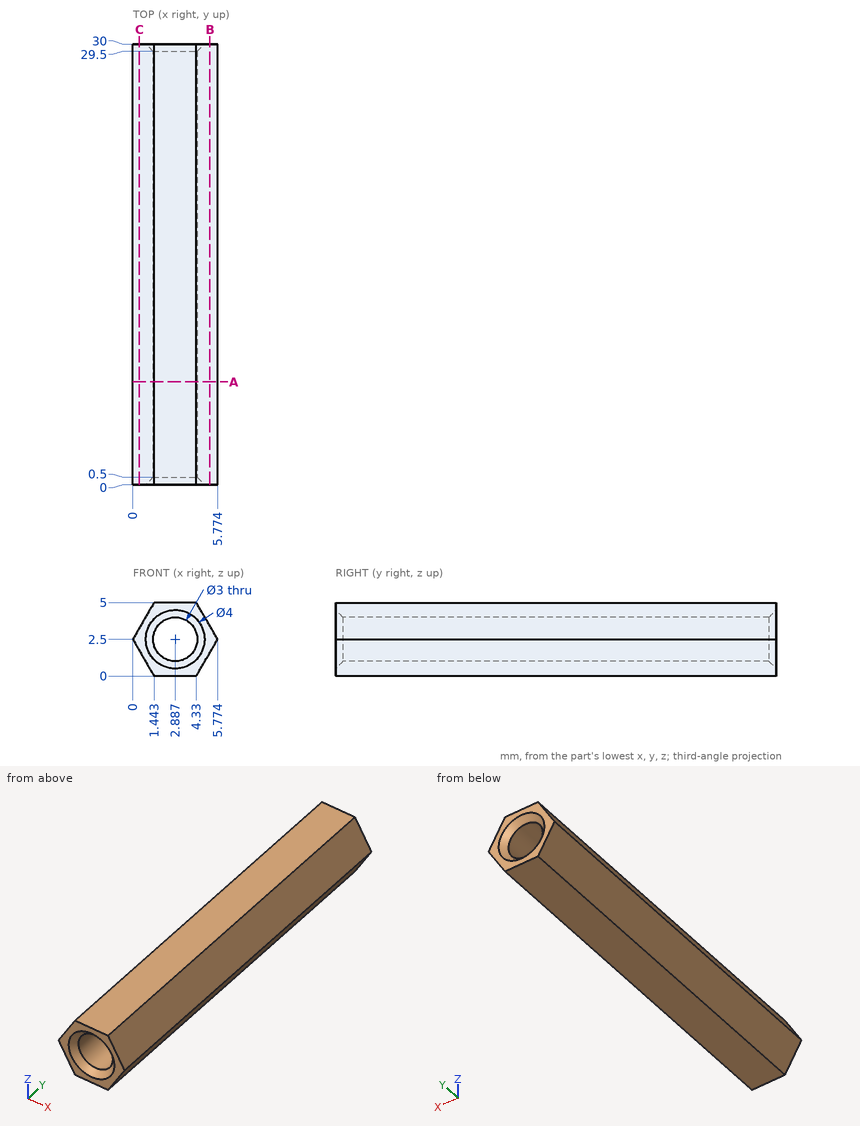
Input: dimensioned drawing with shaded views. Units: mm. Origin: part minimum x, y, z. Round coordinates to 2 decimals unless told otherwise and drop trailing zeros. Order: outer loops, then holes, each group sorted by start corner. A loop starts at its lowest first (then second) coordinate and runs counter-clockwise, first axis right, second up. Notation, with made-up numbers: M 61.5,-24.5 L 109.5,-24.5 A22 cw 109.5,-12.5 Z; hole C 30.5,-21 d5. An arc over 180 degrees is marked long. Use one line per item in the form item = value. Start each with the question number.
Q1. Cut plane A-A (y = 7). Return loops of the section in (x, z), and give its area (3 significant figures).
Q2. Cut plane C-C (x = 0.45). Return loops of the section in (y, z).
Q3. Material intervals for line 1 (Z direction, x = 2.75, y = 27); line 2 (Z direction, x = 2.35, y = 28.25); line 3 (X direction, y = 4, z = 3.25) (1 decimal), sorted ascending. Write a range as [from, to].
Q4. Pin query (flat end, axial travel): pin 1 Ø1 at (x, y) = (5, 4.5) entering from -Z (1 decimal); pin 2 Ø1.8 at (x, z) = (2.89, 2.5) entering from -Y; pin 3 Ø1.5 at (y, z) = (14, 3) entering from -X; pin 4 Ø1.5 at (y, z) = (11, 1.5) entering from -X (1 decimal). Return the tip coordinate at first contact, or that it passes through.
Q5. Cut plane B-B (x = 5.25). Return loops of the section in (y, z).
Geometry results:
q1.outline = M 0,2.5 L 1.44,0 L 4.33,0 L 5.77,2.5 L 4.33,5 L 1.44,5 Z; hole C 2.89,2.5 d3
q1.area = 14.6 mm^2
q2.outline = M 0,1.72 L 30,1.72 L 30,3.28 L 0,3.28 Z
q3.line_1 = [0, 1.01], [3.99, 5]
q3.line_2 = [0, 1.1], [3.9, 5]
q3.line_3 = [0.4, 1.6], [4.2, 5.3]
q4.pin_1 = 0.3
q4.pin_2 = through
q4.pin_3 = 0
q4.pin_4 = 0.1
q5.outline = M 0,1.59 L 30,1.59 L 30,3.41 L 0,3.41 Z
